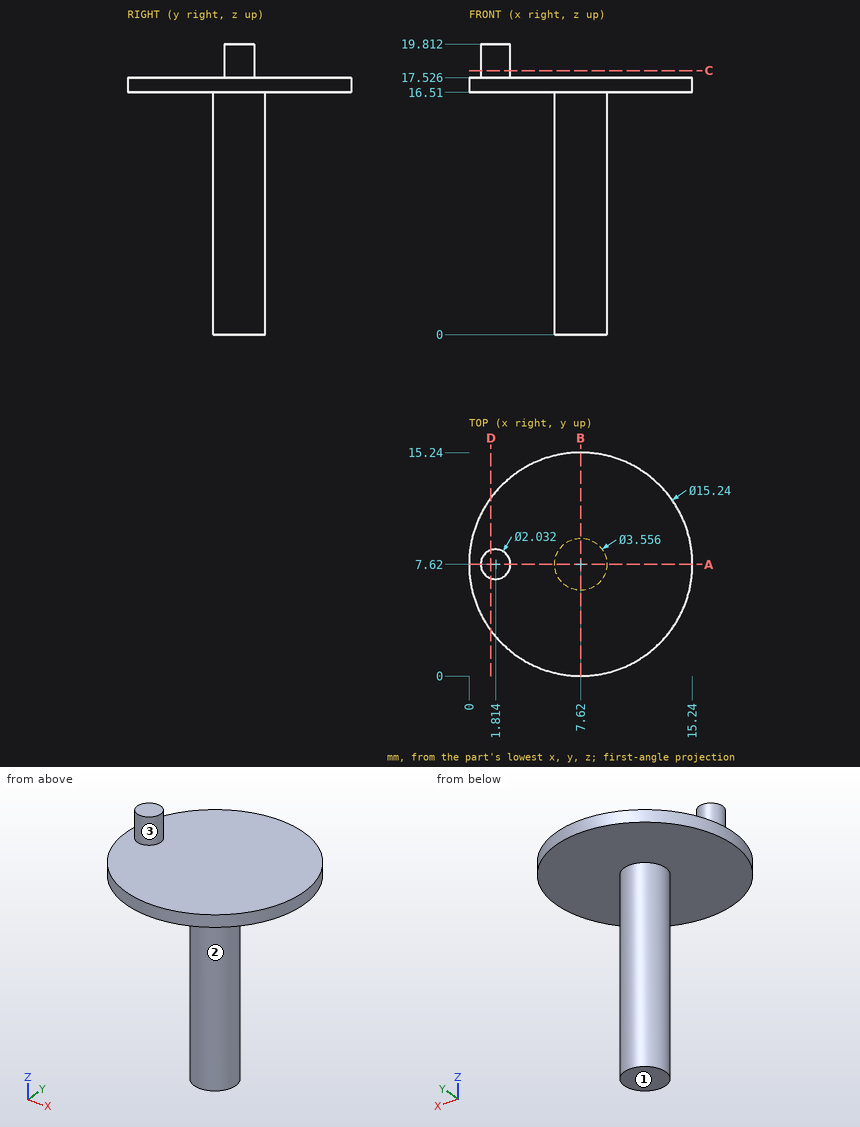
Source: three-view drawing plus pictorial views. Frame: mm from the lowest corner of the part. A direction names the side the tool comes from. Give positions to 0.01 mm unless a question says otherwise; leave off trailing zeros. Write each loop counter-clockwise with the first axis right and the second up, starting at its lowest first coordinate (ties: lowest second). Pieces come first, ordered by that corner, then holes.
(1) Cut plane D-D, the plane x = 1.5. Return loops of the section in (y, z).
(2) Access query for the marked faces 1, 2 and 3. Directions: +Z, -Z, +X, -X, +Y, -Y. A direction counts if a zero-diameter tool reaches every point of the face in a straight line with its end or side. Return the directions, or none.
(3) Cut plane C-C, the plane z = 18. Return loops of the section in (x, y).
(4) First-contact query: P1, Ø1, axis at x = 8.5, z = 14.5, coming from the +Y side; P2, Ø1, axis at y = 7.5, z = 14.5, coming from the -X side; P3, Ø4, axis at x = 7.5, y = 3, coming from the +Z side; P4, Ø2, axis at x = 4.5, z = 7, coming from the +Y side (3 decimals). Flat tips, straight axial feed; report the tip coordinate or a pass-through.
(5) Cut plane B-B, the plane x = 7.62. Return loops of the section in (y, z), then the cut area to 3 significant figures.
(6) Cut plane A-A, the plane y = 7.62. Return loops of the section in (x, z).
(7) Ray query, line 1 (Z direction, x = 5.5, y = 2.25); line 2 (X direction, y = 7.5, z = 1); line 3 (Z direction, x = 6.5, y = 6.75). Return the intervals inside material, ascending.
Values follow:
1. outline: (3.08, 16.51) - (12.16, 16.51) - (12.16, 17.53) - (8.59, 17.53) - (8.59, 19.81) - (6.65, 19.81) - (6.65, 17.53) - (3.08, 17.53) - close
2. face 1: -Z, +X, -X, +Y, -Y
2. face 2: -Z
2. face 3: +Z
3. outline: circle Ø2.03 at (1.81, 7.62)
4. P1: stops at y = 9.36
4. P2: stops at x = 5.84
4. P3: stops at z = 17.53
4. P4: passes through
5. outline: (0, 16.51) - (5.84, 16.51) - (5.84, 0) - (9.4, 0) - (9.4, 16.51) - (15.24, 16.51) - (15.24, 17.53) - (0, 17.53) - close
5. area: 74.2 mm2
6. outline: (0, 16.51) - (5.84, 16.51) - (5.84, 0) - (9.4, 0) - (9.4, 16.51) - (15.24, 16.51) - (15.24, 17.53) - (2.83, 17.53) - (2.83, 19.81) - (0.8, 19.81) - (0.8, 17.53) - (0, 17.53) - close
7. line 1: z = 16.51 to 17.53
7. line 2: x = 5.85 to 9.39
7. line 3: z = 0 to 17.53
